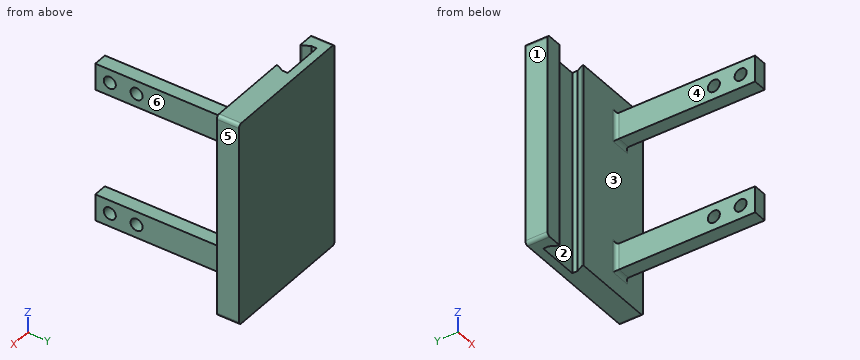
from build123d import *

# Parameters (mm, degrees)
SKETCH2_W           = 50.8
SKETCH2_H           = 76.2
BOSS_EXTRUDE1_DEPTH = 3.175
SKETCH2_5_W         = 6.35
SKETCH2_5_H         = 76.2
SKETCH2_5_W_2       = 5.08
SKETCH2_5_H_2       = 9.906
BOSS_EXTRUDE2_DEPTH = 5.08
SKETCH2_6_W         = 5.08
SKETCH2_6_H         = 4.826
SKETCH2_6_H_2       = 5.08
BOSS_EXTRUDE3_DEPTH = 57.15
SKETCH4_R           = 2.249999945
CUT_EXTRUDE1_DEPTH  = 50.8
FILLET1_R           = 1.27
SKETCH5_W           = 1.3208
SKETCH5_H           = 2.0066
CUT_EXTRUDE2_DEPTH  = 101.6
FILLET2_R           = 0.635


with BuildPart() as part:
    # Sketch2 → Boss-Extrude1 (new body)
    with BuildSketch(Plane(origin=(0, 0, 0), x_dir=(1, 0, 0), z_dir=(0, 1, 0))):
        with Locations((25.4, -38.1)):
            Rectangle(SKETCH2_W, SKETCH2_H)
    extrude(amount=BOSS_EXTRUDE1_DEPTH)

    # Sketch2_5 → Boss-Extrude2 (add)
    # profile 1 of 2: a face of its own
    with BuildSketch(Plane(origin=(0, 0, 0), x_dir=(1, 0, 0), z_dir=(0, 1, 0))):
        with Locations((3.175, -38.1)):
            Rectangle(SKETCH2_5_W, SKETCH2_5_H)
    # profile 2 of 2: a face of its own
    with BuildSketch(Plane(origin=(0, 0, 0), x_dir=(1, 0, 0), z_dir=(0, 1, 0))):
        Polygon((50.8, 0), (19.0754, 0), (19.0754, -38.1), (19.0754, -76.2), (50.8, -76.2), align=None)
        with Locations((38.678980046, -62.970991406)):
            Rectangle(SKETCH2_5_W_2, SKETCH2_5_H_2, mode=Mode.SUBTRACT)
        with Locations((38.678980046, -13.229008594)):
            Rectangle(SKETCH2_5_W_2, SKETCH2_5_H_2, mode=Mode.SUBTRACT)
    extrude(amount=-BOSS_EXTRUDE2_DEPTH)

    # Sketch2_6 → Boss-Extrude3 (add)
    with BuildSketch(Plane(origin=(0, 0, 0), x_dir=(1, 0, 0), z_dir=(0, 1, 0))):
        with Locations((38.678980046, -15.769008594)):
            Rectangle(SKETCH2_6_W, SKETCH2_6_H)
        with Locations((38.678980046, -10.816008594)):
            Rectangle(SKETCH2_6_W, SKETCH2_6_H_2)
        with Locations((38.678980046, -65.383991406)):
            Rectangle(SKETCH2_6_W, SKETCH2_6_H_2)
        with Locations((38.678980046, -60.430991406)):
            Rectangle(SKETCH2_6_W, SKETCH2_6_H)
    extrude(amount=-BOSS_EXTRUDE3_DEPTH)

    # Sketch4 → Cut-Extrude1 (cut)
    with BuildSketch(Plane.ZY.offset(-36.138980046)):
        with Locations((13.229008594, -41.743296244)):
            Circle(SKETCH4_R)
        with Locations((13.229008594, -51.743296056)):
            Circle(SKETCH4_R)
        with Locations((62.970991406, -41.743296244)):
            Circle(SKETCH4_R)
        with Locations((62.970991406, -51.743296056)):
            Circle(SKETCH4_R)
    extrude(amount=-CUT_EXTRUDE1_DEPTH, mode=Mode.SUBTRACT)

    # Fillet1
    fillet1_edges = [part.edges().sort_by_distance(p)[0] for p in [
        (50.8, -0.9525, 0),
        (50.8, -0.9525, 76.2),
        (0, -0.9525, 76.2),
        (38.678980046, -5.08, 18.182008594),
        (38.678980046, -5.08, 8.276008594),
        (36.138980046, -5.08, 13.229008594),
        (41.218980046, -5.08, 13.229008594),
        (36.138980046, -5.08, 62.970991406),
        (38.678980046, -5.08, 67.923991406),
        (41.218980046, -5.08, 62.970991406),
        (38.678980046, -5.08, 58.017991406),
        (0, -0.9525, 0),
    ]]
    fillet(fillet1_edges, radius=FILLET1_R)

    # Sketch5 → Cut-Extrude2 (cut)
    with BuildSketch(Plane(origin=(0, 0, 0), x_dir=(-1, 0, 0), z_dir=(0, 0, -1))):
        with Locations((-19.7358, -1.0033)):
            Rectangle(SKETCH5_W, SKETCH5_H)
        Polygon((-19.0754, -4.532028908), (-19.0754, -2.0066), (-20.3962, -2.0066), align=None)
        with Locations((-5.6896, -1.0033)):
            Rectangle(SKETCH5_W, SKETCH5_H)
        Polygon((-5.0292, -2.0066), (-6.35, -2.0066), (-6.35, -4.532028908), align=None)
    extrude(amount=-CUT_EXTRUDE2_DEPTH, mode=Mode.SUBTRACT)

    # Fillet2
    fillet2_edges = [part.edges().sort_by_distance(p)[0] for p in [
        (6.35, -4.532028908, 38.1),
        (19.0754, -4.532028908, 38.1),
    ]]
    fillet(fillet2_edges, radius=FILLET2_R)


solid = part.part
Verification items for the finished model (mm, model axes). Face numbers are marked on the shaded views. A direction names the side the tool comes from. Give positions to 0.01 mm unless a question says otherwise; leave off trailing zeros. Write each loop counter-clockwise with the first axis right and the second up, starting at its lowest first coordinate (ties: lowest second). Pieces come first, ordered by that corner, then holes. Notation, with made-up numbers: M 31.25,81.25 L 56.25,81.25 A30 ccw 56.25,113.25 Z; hole C -1.5,72 d5. An arc over 180 degrees is marked long. Write item = value, one per line.
(1) Sectioned sample at C-C (z = 63). Record the cut outline in (x, y) (3 decimals), then the cut area to 3 significant figures.
Found:
outline = M 0,-5.08 L 6.35,-5.08 L 6.35,-4.688 A0.635 ccw 6.278,-4.394 L 5.029,-2.007 L 5.029,0 L 20.396,0 L 20.396,-2.007 L 19.148,-4.394 A0.635 ccw 19.075,-4.688 L 19.075,-5.08 L 34.869,-5.08 A1.27 cw 36.139,-6.35 L 36.139,-39.493 L 41.219,-39.493 L 41.219,-6.35 A1.27 cw 42.489,-5.08 L 50.8,-5.08 L 50.8,3.175 L 0,3.175 Z; M 36.139,-57.15 L 41.219,-57.15 L 41.219,-53.993 L 36.139,-53.993 Z; M 36.139,-49.493 L 41.219,-49.493 L 41.219,-43.993 L 36.139,-43.993 Z
area = 566 mm2
(2) Go/stop test with flat-tipped pins: pin 1 Ø8 at (y, z) = (-23.5, 15) entering from +X; pin 2 Ø5 at (y, z) = (-51.74, 62.97) entering from -X; pin 3 Ø5.5 at (x, y) = (40, -22) entering from -Z. Record where each tip stops, or that it passes through.
Found:
pin_1 = 41.22
pin_2 = 36.14
pin_3 = 8.28
(3) Sectioned sample at A-A (y = -18). Record the cut outline in (x, z).
Found:
outline = M 36.14,8.28 L 41.22,8.28 L 41.22,18.18 L 36.14,18.18 Z; M 36.14,58.02 L 41.22,58.02 L 41.22,67.92 L 36.14,67.92 Z
(4) Sectioned sample at D-D (z = 54). Record the cut outline in (x, y) (3 decimals), then the cut area to 3 significant figures.
Found:
outline = M 0,-5.08 L 6.35,-5.08 L 6.35,-4.688 A0.635 ccw 6.278,-4.394 L 5.029,-2.007 L 5.029,0 L 20.396,0 L 20.396,-2.007 L 19.148,-4.394 A0.635 ccw 19.075,-4.688 L 19.075,-5.08 L 50.8,-5.08 L 50.8,3.175 L 0,3.175 Z
area = 346 mm2
(5) Access from +Z, -Z, +X, -X, +Y, -Y to the whole of each face (thin tool, end or side, straight path). Record for the marked faces 4, 5 and 6.
Found:
face_4 = +Z, -Z, -X, -Y
face_5 = +Z, -Z, +X, +Y, -Y
face_6 = +Z, -Z, +X, -Y
(6) Material ranges on line 1 (Y direction, x = 37, z = 65) (3 decimals); line 2 (Z direction, x = 39.5, y = -27); line 3 (Y direction, x = 35, z = 45.5) (3 decimals), recorded low to high.
Found:
line_1 = -57.15 to -52.716, -50.771 to -42.716, -40.771 to 3.175
line_2 = 8.28 to 18.18, 58.02 to 67.92
line_3 = -5.08 to 3.175
(7) Draft check along X on the marked faces 1, 2 and 3. Enter one of: released by +X, released by -X, zero draft, split by the parting line, or undercut.
Found:
face_1 = released by -X
face_2 = undercut
face_3 = zero draft
(8) Sectioned sample at B-B (x = 39.5). Record the cut outline in (y, z) (3 decimals).
Found:
outline = M -57.15,8.276 L -6.35,8.276 A1.27 cw -5.08,7.006 L -5.08,0 L 3.175,0 L 3.175,76.2 L -5.08,76.2 L -5.08,69.194 A1.27 cw -6.35,67.924 L -57.15,67.924 L -57.15,58.018 L -6.35,58.018 A1.27 cw -5.08,56.748 L -5.08,19.452 A1.27 cw -6.35,18.182 L -57.15,18.182 Z; hole C -51.743,13.229 d4.5; hole C -51.743,62.971 d4.5; hole C -41.743,13.229 d4.5; hole C -41.743,62.971 d4.5
